from build123d import *

# Parameters (mm, degrees)
BOSS_EXTRUDE1_DEPTH = 50


with BuildPart() as part:
    # Sketch1 → Boss-Extrude1 (new body)
    with BuildSketch(Plane.XY):
        with BuildLine():
            Line((8, -26.551688605), (8, -18.428571429))
            Line((8, -18.428571429), (5, -18.428571429))
            Line((5, -18.428571429), (5, -21.928571429))
            add(Edge.make_bspline(
                [(5, -21.928571429), (5.024758601, -24.831978652), (4.649789686, -25.256197355), (1.780732191, -25.422029081), (1.5, -25.428571429)],
                knots=[0, 0, 0, 0, 0.274480378, 0.304978198, 0.304978198, 0.304978198, 0.304978198], degree=3))
            add(Edge.make_bspline(
                [(1.5, -25.428571429), (1.487835227, -25.428854924), (1.366303422, -25.431501338), (1.24618398, -25.432201725), (1.135408239, -25.428571429)],
                knots=[0.304978198, 0.304978198, 0.304978198, 0.304978198, 0.306299739, 0.318193606, 0.318193606, 0.318193606, 0.318193606], degree=3))
            Line((1.135408239, -25.428571429), (-2, -25.428571429))
            Line((-2, -25.428571429), (-2, -28.428571429))
            Line((-2, -28.428571429), (6.375219325, -28.428571429))
            add(Edge.make_bspline(
                [(8.000000018, -26.592463548), (7.991060741, -28.414640159), (6.375219325, -28.428571429)],
                knots=[0.011004644, 0.011004644, 0.011004644, 1, 1, 1], degree=2))
            Line((8, -26.592463548), (8, -26.551688605))
        make_face()
    extrude(amount=BOSS_EXTRUDE1_DEPTH)


solid = part.part
Here's how the part is built. I have some questions about the finished solid (model axes, mm). A direction names the side the tool comes from. Round coordinates to 2 decimals unless told otherwise and drop trailing zeros. Order: outer loops, then holes, each group sorted by start corner. A loop starts at its lowest first (then second) coordinate and runs counter-clockwise, first axis right, second up. Notation, with made-up numbers: M 65,79.5 L 77,79.5 A24 cw 77,115.5 Z; hole C -36,59 d9. An arc over 180 degrees is marked long. Return JSON: item names as keys, results as strings. Group by question number.
1. If we section it at A-A on x = -1: List the corners of the cut face in (y, z) for me, then the cut area to 3 significant figures.
2. I'm going to push flat-ended pins straight in: pin 1 Ø1.6 at (x, z) = (-0.5, 31.5) entering from +Y; pin 2 Ø1 at (y, z) = (-22.5, 23.5) entering from -X. Where does each tip first touch, or does it pass through?
3. Please list where these lines run through material, in increasing order: probe 1 along X at (y, z) = (-21.75, 14); probe 2 along Y at (x, z) = (0, 42); probe 3 along X at (y, z) = (-26.75, 26.5).
4. If we section it at B-B on y = -20: List the corners of the cut face in (x, z) for me, then the cut area to 3 significant figures.
5. On a 3-axis mill with a long thin cutter (end or side, diameter ignored), from which of +Z, -Z, +X, -X, +Y, -Y can I reach the whole of each face in a straight line? I mean faces 1 (the face through (7, -18.429, 25)), 2 (the face through (5, -20, 25)). Say none if no direction works.
Reply:
{
 "1": {"outline": "M -28.43,0 L -25.43,0 L -25.43,50 L -28.43,50 Z", "area": "150 mm^2"},
 "2": {"pin 1": "y = -25.43", "pin 2": "x = 4.98"},
 "3": {"probe 1": "5 to 8", "probe 2": "-28.43 to -25.43", "probe 3": "-2 to 8"},
 "4": {"outline": "M 5,0 L 8,0 L 8,50 L 5,50 Z", "area": "150 mm^2"},
 "5": {"face 1": "+Z, -Z, +X, -X, +Y", "face 2": "+Z, -Z, -X, +Y"}
}
